Read the model definition and answer for the solid it produces. Units are mm, in the model's axes. Face numbers are marked on the shaded views. Coordinates: 2 decimals unless noted, no trailing zeros. Write each loop counter-clockwise with the first axis right and the second up, starting at its lowest first coordinate (ties: lowest second). Pieces come first, ordered by that corner, then holes. Notation, with made-up numbers: (86, -26.5) -> (136, -26.5) arc R25 ccw to (136, 9.5) -> close; hole circle Ø5 at (74.5, 72). An arc over 180 degrees is marked (long way). Answer in a Markdown table with one row per item. Add a question column.
Item 1: For a pull along Y with two mould halves and no side action, classify the marked faces 1, 2 and 3 as +Y half, -Y half, draft (parallel to the pull), parting line (faces both ways), or undercut.
Item 2: Straight lines are drawn through the part: line 1 (Y direction, x = -12.7, z = 2.25); line 2 (Y direction, x = -11.5, z = 6.75); line 3 (X direction, y = 14.5, z = 2.5). For each, find the intervals that lie inside material, in ascending order. Write a range as from..to.
Item 3: Section B-B on y = -12.7 is taken. Write down the section's boundary in (x, z).
Item 4: Section A-A on x = 0 is taken. Write down the section's boundary in (y, z), then the cut area to 3 significant figures.
Item 5: Section C-C on z = 3.75 is taken. Write down the section's boundary in (x, y).
```python
from build123d import *

# Parameters (mm, degrees)
F0_W     = 50.8
F0_H     = 50.8
F0_R     = 2.794
F0_R_2   = 4.318
F1_DEPTH = 7.62


with BuildPart() as f1:
    # F0 (on Top) → F1 (new body)
    with BuildSketch(Plane.XY):
        Rectangle(F0_W, F0_H)
        with Locations((-12.7, -12.7)):
            Circle(F0_R, mode=Mode.SUBTRACT)
        Circle(F0_R_2, mode=Mode.SUBTRACT)
        with Locations((12.7, -12.7)):
            Circle(F0_R, mode=Mode.SUBTRACT)
        with Locations((-12.7, 12.7)):
            Circle(F0_R, mode=Mode.SUBTRACT)
        with Locations((12.7, 12.7)):
            Circle(F0_R, mode=Mode.SUBTRACT)
    extrude(amount=F1_DEPTH)


solid = f1.part
```
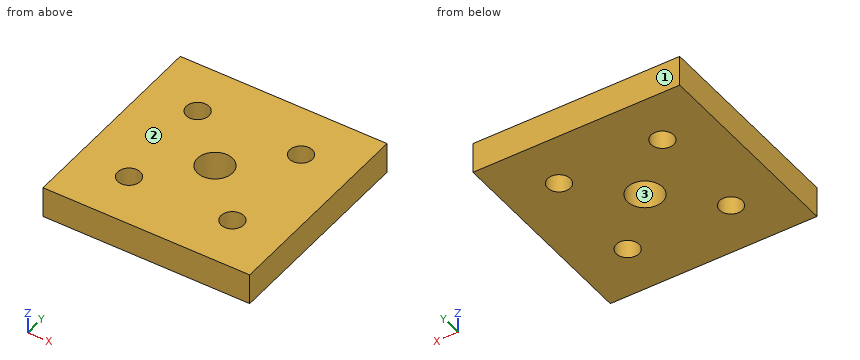
Results below:
| question | item | result |
|---|---|---|
| 1 | face 1 | +Y half |
| 1 | face 2 | draft |
| 1 | face 3 | undercut |
| 2 | line 1 | y = -25.4..-15.49, -9.91..9.91, 15.49..25.4 |
| 2 | line 2 | y = -25.4..-15.22, -10.18..10.18, 15.22..25.4 |
| 2 | line 3 | x = -25.4..-14.84, -10.56..10.56, 14.84..25.4 |
| 3 | outline | (-25.4, 0) -> (-15.49, 0) -> (-15.49, 7.62) -> (-25.4, 7.62) -> close; (-9.91, 0) -> (9.91, 0) -> (9.91, 7.62) -> (-9.91, 7.62) -> close; (15.49, 0) -> (25.4, 0) -> (25.4, 7.62) -> (15.49, 7.62) -> close |
| 4 | outline | (-25.4, 0) -> (-4.32, 0) -> (-4.32, 7.62) -> (-25.4, 7.62) -> close; (4.32, 0) -> (25.4, 0) -> (25.4, 7.62) -> (4.32, 7.62) -> close |
| 4 | area | 321 mm2 |
| 5 | outline | (-25.4, -25.4) -> (25.4, -25.4) -> (25.4, 25.4) -> (-25.4, 25.4) -> close; hole circle Ø5.59 at (-12.7, -12.7); hole circle Ø5.59 at (-12.7, 12.7); hole circle Ø8.64 at (0, 0); hole circle Ø5.59 at (12.7, -12.7); hole circle Ø5.59 at (12.7, 12.7) |
